Geometry: final body of the model. Coordinates: model frame, mm. Face numbers are marked on the shaded views. A direction names the side the tool comes from. Give positions to 0.01 mm unless a question says otherwise; leave off trailing zeros. Write each loop counter-clockwise with the first axis right and the second up, starting at its lowest first coordinate (ties: lowest second). Pieces come first, ordered by that corner, then holes.
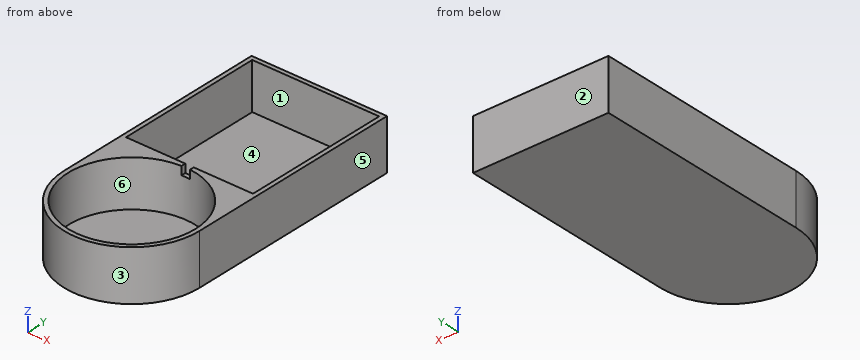
```python
from build123d import *

# Parameters (mm, degrees)
F0_W     = 101.6
F0_H     = 165.1
F1_DEPTH = 38.1
F2_R     = 47.625
F3_DEPTH = 34.925
F4_W     = 6.35
F4_H     = 6.35
F5_DEPTH = 50.8
F6_W     = 95.25
F6_H     = 111.125
F7_DEPTH = 34.925


with BuildPart() as f1:
    # F0 (on Top) → F1 (new body)
    with BuildSketch(Plane.XY):
        with BuildLine():
            Line((50.8, 0), (-50.8, 0))
            ThreePointArc((-50.8, 0), (0, -50.8), (50.8, 0))
        make_face()
        with Locations((0, 82.55)):
            Rectangle(F0_W, F0_H)
    extrude(amount=F1_DEPTH)

    # F2 (on face) → F3 (cut)
    with BuildSketch(Plane.XY.offset(38.1)):
        Circle(F2_R)
    extrude(amount=-F3_DEPTH, mode=Mode.SUBTRACT)

    # F4 (on Front) → F5 (cut)
    with BuildSketch(Plane.XZ):
        with Locations((0, 34.925)):
            Rectangle(F4_W, F4_H)
    extrude(amount=-F5_DEPTH, mode=Mode.SUBTRACT)

    # F6 (on face) → F7 (cut)
    with BuildSketch(Plane.XY.offset(38.1)):
        with Locations((0, 106.3625)):
            Rectangle(F6_W, F6_H)
    extrude(amount=-F7_DEPTH, mode=Mode.SUBTRACT)


solid = f1.part
```
Item 1: Reachability of the marked faces 5 and 6 from +Z, -Z, +X, -X, +Y, -Y: full face, straight path, thin tool, end or side. Return the list, or none.
Found:
face 5: +Z, -Z, +X, +Y, -Y
face 6: +Z
Item 2: Section D-D, the plane x = 0. Return the cut outline in (y, z) (3 decimals), plus the area to 3 significant figures.
Found:
outline: (-50.8, 0) - (165.1, 0) - (165.1, 38.1) - (161.925, 38.1) - (161.925, 3.175) - (50.8, 3.175) - (50.8, 31.75) - (47.625, 31.75) - (47.625, 3.175) - (-47.625, 3.175) - (-47.625, 38.1) - (-50.8, 38.1) - close
area: 998 mm2
Item 3: Section B-B, the plane z = 36. Return the cut outline in (x, y) (3 decimals), plus the area to 3 significant figures.
Found:
outline: (-50.8, 0) arc R50.8 ccw to (50.8, 0) - (50.8, 165.1) - (-50.8, 165.1) - close; hole (-47.625, 50.8) - (-3.175, 50.8) - (-3.175, 47.519) arc R47.625 ccw (long way) to (3.175, 47.519) - (3.175, 50.8) - (47.625, 50.8) - (47.625, 161.925) - (-47.625, 161.925) - close
area: 3,100 mm2
Item 4: Section C-C, the plane y = 150.5. Return the cut outline in (x, z) (3 decimals), plus the area to 3 significant figures.
Found:
outline: (-50.8, 0) - (50.8, 0) - (50.8, 38.1) - (47.625, 38.1) - (47.625, 3.175) - (-47.625, 3.175) - (-47.625, 38.1) - (-50.8, 38.1) - close
area: 544 mm2
Item 5: Pull-direction query (Y, two-part tool) for the marked faces 1, 2, 3 and 4; classes: +Y half, -Y half, draft (parallel to the pull), parting line (faces both ways), or undercut.
Found:
face 1: undercut
face 2: +Y half
face 3: -Y half
face 4: undercut
Item 6: Line query: L1, parallel to Y at x = 0, z = 18 (3 decimals); L2, parallel to X at y = 0, z = 17 (3 decimals); L3, parallel to Z at x = -11, y = 108 (3 decimals). Output: solid intervals per line, ascending.
Found:
L1: y = -50.8 to -47.625, 47.625 to 50.8, 161.925 to 165.1
L2: x = -50.8 to -47.625, 47.625 to 50.8
L3: z = 0 to 3.175
Item 7: Pin query (flat end, axial travel): pin 1 Ø3 at (x, z) = (-17, 25) entering from -Y; pin 2 Ø8 at (x, z) = (-15.5, 11.5) entering from -Y; pin 3 Ø10 at (y, z) = (-15.5, 9) entering from +X. Return the tip coordinate at first contact, or that it passes through.
Found:
pin 1: stops at y = -48.38
pin 2: stops at y = -49.48
pin 3: stops at x = 49.7
Item 8: Section A-A, the plane z = 19. Return the cut outline in (x, y) (3 decimals), plus the area to 3 significant figures.
Found:
outline: (-50.8, 0) arc R50.8 ccw to (50.8, 0) - (50.8, 165.1) - (-50.8, 165.1) - close; hole circle Ø95.25 at (0, 0); hole (-47.625, 50.8) - (47.625, 50.8) - (47.625, 161.925) - (-47.625, 161.925) - close
area: 3,120 mm2
